Read the model definition and answer for the solid it produces. Units are mm, in the model's axes. A direction names the side the tool comes from. Give positions to 0.01 mm unless a question says otherwise; leave off trailing zeros. Order: outer loops, then holes, each group sorted by start corner. A loop starts at its lowest first (then second) coordinate and runs counter-clockwise, first axis right, second up.
Item 1: A cutting plane is placed at D-D (y = 9). Write down the section's boundary in (x, z).
Item 2: The mould has two halves that part along X. Classify faces 1 (the face through (-40, 0, 10)), 2 (the face through (-1, -28, 11)), 3 (the face through (-1, 0, 0)): +X half, -X half, draft (parallel to the pull), parting line (faces both ways), or undercut.
Item 3: Find the intervals of material crossed by line 1 along Y through (x, z) = (9, 4.5); line 2 along X through (y, z) = (9, 5); line 3 along Z through (x, y) = (1, -14), in increasing order.
Item 4: A cutting plane is placed at B-B (z = 4.75). Write down the section's boundary in (x, y).
Item 5: Given pin 1 Ø10 at (x, y) = (-29.5, 14) entering from +Z, flat-ended and moving along its own axis, determine where the tip first touches the part or whether it passes through.
Item 6: A cutting plane is placed at A-A (y = -16). Write down the section's boundary in (x, z).
Item 7: Which of the six approach directions +Z, -Z, +X, -X, +Y, -Y give full straight-line access (tool end or side, diameter ignored) to faces 4 (the face through (-1, 0, 2)), 5 (the face through (-1, 30, 10)), 6 (the face through (40, 0, 10)), 7 (the face through (39.01, 22.41, 6.26)), 8 (the face through (-39, -14, 12))?
Item 8: A cutting plane is placed at C-C (x = 32). Write down the section's boundary in (y, z).
from build123d import *

# Parameters (mm, degrees)
SKETCH_W        = 80
SKETCH_H        = 60
PAD_DEPTH       = 20
SKETCH001_W     = 76
SKETCH001_H     = 56
POCKET_DEPTH    = 18
SKETCH002_W     = 18
SKETCH002_H     = 5
POCKET001_DEPTH = 5
SKETCH003_R     = 4
SKETCH003_R_2   = 3
POCKET002_DEPTH = 5


with BuildPart() as part:
    # Sketch → Pad (new body)
    with BuildSketch(Plane.XY):
        Rectangle(SKETCH_W, SKETCH_H)
    extrude(amount=PAD_DEPTH)

    # Sketch001 (on Face6 of Pad) → Pocket (cut)
    with BuildSketch(Plane.XY.offset(20)):
        Rectangle(SKETCH001_W, SKETCH001_H)
    extrude(amount=-POCKET_DEPTH, mode=Mode.SUBTRACT)

    # Sketch002 (on Face2 of Pocket) → Pocket001 (cut)
    with BuildSketch(Plane(origin=(-40, 0, 0), x_dir=(0, -1, 0), z_dir=(-1, 0, 0))):
        with Locations((14, 9.5)):
            Rectangle(SKETCH002_W, SKETCH002_H)
    extrude(amount=-POCKET001_DEPTH, mode=Mode.SUBTRACT)

    # Sketch003 (on Face3 of Pocket001) → Pocket002 (cut)
    with BuildSketch(Plane.YZ.offset(40)):
        with Locations((20.562784, 9.80915)):
            Circle(SKETCH003_R)
        with Locations((-20.052979, 9.809152)):
            Circle(SKETCH003_R_2)
    extrude(amount=-POCKET002_DEPTH, mode=Mode.SUBTRACT)


solid = part.part
Response values:
1. outline: (-40, 0) - (40, 0) - (40, 20) - (38, 20) - (38, 2) - (-38, 2) - (-38, 20) - (-40, 20) - close
2. face 1: -X half
2. face 2: undercut
2. face 3: draft
3. line 1: y = -30 to -28, 28 to 30
3. line 2: x = -40 to -38, 38 to 40
3. line 3: z = 0 to 2
4. outline: (-40, -30) - (40, -30) - (40, 30) - (-40, 30) - close; hole (-38, -28) - (38, -28) - (38, 28) - (-38, 28) - close
5. pin 1: stops at z = 2
6. outline: (-40, 0) - (40, 0) - (40, 20) - (38, 20) - (38, 2) - (-38, 2) - (-38, 7) - (-40, 7) - close; (-40, 12) - (-38, 12) - (-38, 20) - (-40, 20) - close
7. face 4: +Z
7. face 5: +Z, -Z, +X, -X, +Y
7. face 6: +Z, -Z, +X, +Y, -Y
7. face 7: +X
7. face 8: -X
8. outline: (-30, 0) - (30, 0) - (30, 20) - (28, 20) - (28, 2) - (-28, 2) - (-28, 20) - (-30, 20) - close
